```python
from build123d import *

# Parameters (mm, degrees)
EXTRUDE_1_DEPTH     = 2
EXTRUDE_2_DEPTH     = 27
SKETCH_4_R          = 3.227350269
CUT_EXTRUDE_1_DEPTH = 2
CUT_EXTRUDE_2_DEPTH = 0.5
CUT_EXTRUDE_3_DEPTH = 1
CUT_EXTRUDE_4_DEPTH = 34.256578297
SKETCH_8_W          = 12
SKETCH_8_H          = 1
EXTRUDE_3_DEPTH     = 1.6


with BuildPart() as part:
    # 草图1 → 凸台-拉伸1 (new body)
    with BuildSketch(Plane.XY):
        with BuildLine():
            Line((-5.5, -5), (5.5, -5))
            ThreePointArc((5.5, -5), (5.853553391, -4.853553391), (6, -4.5))
            Line((6, -4.5), (6, 4.5))
            ThreePointArc((6, 4.5), (5.853553391, 4.853553391), (5.5, 5))
            Line((5.5, 5), (4, 5))
            Line((4, 5), (4, 0))
            ThreePointArc((4, 0), (0, -4), (-4, 0))
            Line((-4, 0), (-4, 5))
            Line((-4, 5), (-5.5, 5))
            ThreePointArc((-5.5, 5), (-5.853553391, 4.853553391), (-6, 4.5))
            Line((-6, 4.5), (-6, -4.5))
            ThreePointArc((-6, -4.5), (-5.853553391, -4.853553391), (-5.5, -5))
        make_face()
        with BuildLine():
            Line((-8, -3), (-13.875, -3))
            Line((-13.875, -3), (-13.875, -9))
            Line((-13.875, -9), (16, -9))
            Line((16, -9), (16, -7))
            Line((16, -7), (-11.875, -7))
            Line((-11.875, -7), (-11.875, -5))
            Line((-11.875, -5), (-8, -5))
            Line((-8, -5), (-5.5, -5))
            ThreePointArc((-5.5, -5), (-5.853553391, -4.853553391), (-6, -4.5))
            Line((-6, -4.5), (-6, 4.5))
            ThreePointArc((-6, 4.5), (-5.853553391, 4.853553391), (-5.5, 5))
            Line((-5.5, 5), (-4, 5))
            Line((-4, 5), (4, 5))
            Line((4, 5), (5.5, 5))
            ThreePointArc((5.5, 5), (5.853553391, 4.853553391), (6, 4.5))
            Line((6, 4.5), (6, -4.5))
            ThreePointArc((6, -4.5), (5.853553391, -4.853553391), (5.5, -5))
            Line((5.5, -5), (8, -5))
            Line((8, -5), (16, -5))
            Line((16, -5), (16, -3))
            Line((16, -3), (8, -3))
            Line((8, -3), (8, 7))
            Line((8, 7), (-8, 7))
            Line((-8, 7), (-8, -3))
        make_face()
        Polygon((-11.875, -7), (16, -7), (16, -5), (8, -5), (5.5, -5), (-5.5, -5), (-8, -5), (-11.875, -5), align=None)
    extrude(amount=EXTRUDE_1_DEPTH)

    # 草图2 → 凸台-拉伸2 (add)
    with BuildSketch(Plane(origin=(0, 0, 0), x_dir=(-1, 0, 0), z_dir=(0, 0, -1))):
        Polygon((-6, 4.5), (-6, 5), (-5.5, 5), (5.5, 5), (6, 5), (6, 4.5), (6, -4.5), (6, -5), (11.875, -5), (11.875, -7), (-16, -7), (-16, -9), (13.875, -9), (13.875, -3), (8, -3), (8, 7), (-8, 7), (-8, -3), (-16, -3), (-16, -5), (-6, -5), (-6, -4.5), align=None)
    extrude(amount=EXTRUDE_2_DEPTH)

    # 草图4 → 切除-拉伸1 (cut)
    with BuildSketch(Plane.XZ.offset(9)):
        with Locations(Location((11.625, -15.5, 0), (0, 0, 270))):
            Circle(SKETCH_4_R)
    extrude(amount=-CUT_EXTRUDE_1_DEPTH, mode=Mode.SUBTRACT)

    # 草图5 → 切除-拉伸2 (cut)
    with BuildSketch(Plane(origin=(0, -3, 0), x_dir=(1, 0, 0), z_dir=(0, 1, 0))):
        Polygon((11.625, 18.675426481), (8.875, 17.08771324), (8.875, 13.91228676), (11.625, 12.324573519), (14.375, 13.91228676), (14.375, 17.08771324), align=None)
    extrude(amount=-CUT_EXTRUDE_2_DEPTH, mode=Mode.SUBTRACT)

    # 草图6 → 切除-拉伸3 (cut)
    with BuildSketch(Plane(origin=(0, -3, 0), x_dir=(1, 0, 0), z_dir=(0, 1, 0))):
        Polygon((8.625, 2.267949192), (11.625, 0.535898385), (14.625, 2.267949192), (14.625, 5.732050808), (11.625, 7.464101615), (8.625, 5.732050808), align=None)
    extrude(amount=-CUT_EXTRUDE_3_DEPTH, mode=Mode.SUBTRACT)

    # 草图7 → 切除-拉伸4 (cut, through all)
    with BuildSketch(Plane(origin=(0, -4, 0), x_dir=(1, 0, 0), z_dir=(0, 1, 0))):
        with BuildLine():
            ThreePointArc((13.225, 4), (12.75637085, 5.13137085), (11.625, 5.6))
            Line((11.625, 5.6), (11.625, 2.4))
            ThreePointArc((11.625, 2.4), (12.75637085, 2.86862915), (13.225, 4))
        make_face()
        with BuildLine():
            Line((11.625, 2.4), (11.625, 5.6))
            ThreePointArc((11.625, 5.6), (10.025, 4), (11.625, 2.4))
        make_face()
    extrude(amount=-CUT_EXTRUDE_4_DEPTH, mode=Mode.SUBTRACT)

    # 草图8 → 凸台-拉伸3 (add)
    with BuildSketch(Plane(origin=(0, 0, -27), x_dir=(-1, 0, 0), z_dir=(0, 0, -1))):
        with Locations((0, 4.5)):
            Rectangle(SKETCH_8_W, SKETCH_8_H)
    extrude(amount=-EXTRUDE_3_DEPTH)


solid = part.part
```
CAD build for the part. Positions are in the model's coordinates, mm. A direction names the side the tool comes from. Coordinates: 2 decimals unless noted, no trailing zeros. Write each loop counter-clockwise with the first axis right and the second up, starting at its lowest first coordinate (ties: lowest second). Pieces come first, ordered by that corner, then holes.
(1) Flat gauge pins, fed straight in: pin 1 (3 mm diameter, centred on y = 2.5, z = -20.5, fed in from +X); pin 2 (4.5 mm diameter, centred on x = 10.5, z = -14, fed in from +Y); pin 3 (4 mm diameter, centred on x = 11.625, z = -15.5, fed in from +Y). Where does each tip first touch, or does it go through?
(2) Cut at A-A, the plane y = 1.75. List the corners of the cut face in (x, z), and give its area (3 significant figures).
(3) Cut at B-B, the plane z = -15.5. List the corners of the cut face in (x, y) (3 decimals).
(4) Cut at C-C, the plane x = -10.5. List the corners of the cut face in (y, z), and give its area (3 significant figures).
(5) Drill centre lines: probe 1 along Y at (x, z) = (-10.75, -25); probe 2 along Y at (x, z) = (-1.5, -12); probe 3 along X at (y, z) = (-8.6, -15.5) (3 decimals). Where is each one in solid material? Low to high.
(6) Cut at D-D, the plane x = 0. List the corners of the cut face in (y, z), and give its area (3 significant figures).
(7) Two-plate mould, pull along Y, no slides. Class faces 4 (the face through (11, -5, -13)), 5 (the face through (12, -3, -12)), 6 (the face through (-13.875, -6, -12)): +Y half, -Y half, draft (parallel to the pull), parting line (faces both ways), or undercut.
(8) 3-axis set-ups, long thin cutter, end or side, ignore diameter. For faces 1 (the face through (-11.875, -6, -13)), 2 (the face through (-8, 2, -12)), 3 (the face through (0.1, 4.5, -25.4)): which of +Z, -Z, +X, -X, +Y, -Y reach the whole face in a straight line?
Geometry says:
1. pin 1: stops at x = 8
1. pin 2: stops at y = -3
1. pin 3: stops at y = -3.5
2. outline: (-8, -27) - (-6, -27) - (-6, 0) - (-4, 0) - (-4, 2) - (-8, 2) - close; (4, 0) - (6, 0) - (6, -27) - (8, -27) - (8, 2) - (4, 2) - close
2. area: 124 mm2
3. outline: (-13.875, -9) - (8.398, -9) - (8.398, -7) - (-11.875, -7) - (-11.875, -5) - (-6, -5) - (-6, 5) - (6, 5) - (6, -5) - (16, -5) - (16, -3) - (14.375, -3) - (14.375, -3.5) - (8.875, -3.5) - (8.875, -3) - (8, -3) - (8, 7) - (-8, 7) - (-8, -3) - (-13.875, -3) - close; (14.852, -9) - (16, -9) - (16, -7) - (14.852, -7) - close
4. outline: (-9, -27) - (-7, -27) - (-7, 0) - (-5, 0) - (-5, -27) - (-3, -27) - (-3, 2) - (-9, 2) - close
4. area: 120 mm2
5. probe 1: y = -9 to -7, -5 to -3
5. probe 2: y = -9 to -7, 5 to 7
5. probe 3: x = -13.875 to 8.398, 14.852 to 16
6. outline: (-9, -27) - (-7, -27) - (-7, 0) - (-4, 0) - (-4, 2) - (-9, 2) - close; (4, -27) - (7, -27) - (7, 2) - (5, 2) - (5, -25.4) - (4, -25.4) - close
6. area: 124 mm2
7. face 4: undercut
7. face 5: +Y half
7. face 6: draft
8. face 1: -Z, +X
8. face 2: +Z, -Z, -X, +Y
8. face 3: none
